Geometry check sheet. Reference: the model listing, model coordinates, mm. A direction names the side the tool comes from. Coordinates: 2 decimals unless noted, no trailing zeros. Write each loop counter-clockwise with the first axis right and the second up, starting at its lowest first coordinate (ties: lowest second). Pieces come first, ordered by that corner, then holes. Notation, with made-up numbers: (62, 20.25) -> (108, 20.25) arc R18 ccw to (108, 32.25) -> close; hole circle Ø4 at (37, -21.75). An arc over 180 degrees is marked (long way). Answer in a Markdown table with one row per item. Add a question column.
1. Cross-section at C-C on x = 0. Record the cut outline in (y, z), and give its area (3 significant figures).
2. Set-up check for faces 5 (the flat face through (14, 0, 0)), 6 (the flat face through (-11.341, 0, 1)): record each of +Z, -Z, +X, -X, +Y, -Y from which the full face is reachable in a straight line by a thin tool's end or side.
3. Depth check by flat-ended pin: P1, Ø12, axis at x = -1.5, y = -11, coming from the +Z side. Enter the tip coordinate at first touch or a pass-through.
4. Cross-section at D-D on y = 17. Record the cut outline in (x, z).
5. Mould release check, pull along Y, two halves, no side actions. Record for faces 1 (the flat face through (14, 0, 1.524)), 2 (the cylindrical face through (-2.868, 21.847, 0.751)), 3 (the cylindrical face through (-9.9, -13, 0.8)), 4 (the flat face through (0, 14.351, 1)): pulls with the +Y half, pulls with the -Y half, needs draft (parallel to the pull), parting line crosses it, or undercut.
6. Cross-section at B-B on z = 1.1. Record the cut outline in (x, y) (1 decimal).
7. Cross-section at A-A on y = 0. Record the cut outline in (x, z).
8. Scan lines: L1, parallel to Y at x = 9.5, z = 0.7; L2, parallel to X at y = -12.5, z = 1.15; L3, parallel to X at y = 3.5, z = 1. Record each from-to range of solid material in increasing order. Write a range as from..to.
```python
from build123d import *

# Parameters (mm, degrees)
SKETCH1_R      = 22.0345
SKETCH1_W      = 22.6822
SKETCH1_H      = 28.702
EXTRUDE1_DEPTH = 1.524
FILLET1_R      = 4.7625


with BuildPart() as part:
    # Sketch1 → Extrude1 (new body)
    with BuildSketch(Plane.XY):
        Circle(SKETCH1_R)
        Rectangle(SKETCH1_W, SKETCH1_H, mode=Mode.SUBTRACT)
    extrude(amount=EXTRUDE1_DEPTH)

    # Fillet1
    fillet1_edges = [part.edges().sort_by_distance(p)[0] for p in [
        (-11.3411, 14.351, 0.762),
        (-11.3411, -14.351, 0.762),
        (11.3411, -14.351, 0.762),
        (11.3411, 14.351, 0.762),
    ]]
    fillet(fillet1_edges, radius=FILLET1_R)


solid = part.part
```
Results found:
| question | item | result |
|---|---|---|
| 1 | outline | (-22.03, 0) -> (-14.35, 0) -> (-14.35, 1.52) -> (-22.03, 1.52) -> close; (14.35, 0) -> (22.03, 0) -> (22.03, 1.52) -> (14.35, 1.52) -> close |
| 1 | area | 23.4 mm^2 |
| 2 | face 5 | -Z, +X, -X, +Y, -Y |
| 2 | face 6 | +Z, -Z |
| 3 | P1 | stops at z = 1.52 |
| 4 | outline | (-14.02, 0) -> (14.02, 0) -> (14.02, 1.52) -> (-14.02, 1.52) -> close |
| 5 | face 1 | needs draft |
| 5 | face 2 | parting line crosses it |
| 5 | face 3 | undercut |
| 5 | face 4 | undercut |
| 6 | outline | circle Ø44.1 at (0, 0); hole (-11.3, -9.6) arc R4.8 ccw to (-6.6, -14.4) -> (6.6, -14.4) arc R4.8 ccw to (11.3, -9.6) -> (11.3, 9.6) arc R4.8 ccw to (6.6, 14.4) -> (-6.6, 14.4) arc R4.8 ccw to (-11.3, 9.6) -> close |
| 7 | outline | (-22.03, 0) -> (-11.34, 0) -> (-11.34, 1.52) -> (-22.03, 1.52) -> close; (11.34, 0) -> (22.03, 0) -> (22.03, 1.52) -> (11.34, 1.52) -> close |
| 8 | L1 | y = -19.88..-13.35, 13.35..19.88 |
| 8 | L2 | x = -18.15..-10.35, 10.35..18.15 |
| 8 | L3 | x = -21.75..-11.34, 11.34..21.75 |
